from build123d import *

# Parameters (mm, degrees)
F0_W      = 1778
F0_H      = 279.4
F1_DEPTH  = 25.4
F2_W      = 1727.2
F2_H      = 228.6
F3_DEPTH  = 25.401
F4_W      = 279.4
F4_H      = 279.4
F5_DEPTH  = 25.4
F6_W      = 127
F6_H      = 25.4
F7_DEPTH  = 25.4
F8_W      = 127
F8_H      = 25.4
F9_DEPTH  = 25.4
F10_W     = 127
F10_H     = 25.4
F11_DEPTH = 25.4
F12_W     = 127
F12_H     = 25.4
F13_DEPTH = 25.4


with BuildPart() as f1:
    # F0 (on Top) → F1 (new body)
    with BuildSketch(Plane.XY):
        Rectangle(F0_W, F0_H)
    extrude(amount=F1_DEPTH)

    # F2 (on face) → F3 (cut, through all)
    with BuildSketch(Plane.XY.offset(25.4)):
        Rectangle(F2_W, F2_H)
    extrude(amount=-F3_DEPTH, mode=Mode.SUBTRACT)

    # F4 (on Top) → F5 (join)
    with BuildSketch(Plane.XY):
        Rectangle(F4_W, F4_H)
    extrude(amount=F5_DEPTH)

    # F6 (on face) → F7 (join)
    with BuildSketch(Plane(origin=(-889, 0, 0), x_dir=(0, -1, 0), z_dir=(-1, 0, 0))):
        with Locations((0, 12.7)):
            Rectangle(F6_W, F6_H)
    extrude(amount=F7_DEPTH)

    # F8 (on face) → F9 (join)
    with BuildSketch(Plane(origin=(863.6, 0, 0), x_dir=(0, -1, 0), z_dir=(-1, 0, 0))):
        with Locations((0, 12.7)):
            Rectangle(F8_W, F8_H)
    extrude(amount=F9_DEPTH)

    # F10 (on face) → F11 (join)
    with BuildSketch(Plane.YZ.offset(889)):
        with Locations((0, 12.7)):
            Rectangle(F10_W, F10_H)
    extrude(amount=F11_DEPTH)

    # F12 (on face) → F13 (join)
    with BuildSketch(Plane.YZ.offset(-863.6)):
        with Locations((0, 12.7)):
            Rectangle(F12_W, F12_H)
    extrude(amount=F13_DEPTH)


solid = f1.part
Verification items for the finished model (mm, model axes). Coordinates: 2 decimals unless noted, no trailing zeros. Order: outer loops, then holes, each group sorted by start corner. A loop starts at its lowest first (then second) coordinate and runs counter-clockwise, first axis right, second up. Notation, with made-up numbers: (31, -3.75) -> (89, -3.75) arc R15 ccw to (89, 9.25) -> close; hole circle Ø10 at (-21, -27). An arc over 180 degrees is marked (long way). Put each result on its own line as item: value. Start each with the question number.
1. Material ranges on L1, parallel to X at y = 79.5, z = 18.25; L2, parallel to X at y = -21.5, z = 5.25; L3, parallel to Y at x = 687, z = 19, recorded low to high. Write a range as [from, to].
2. Cross-section at A-A, the plane y = -43.5. Record the boundary of the cut face in (x, z), then the cut area to 3 significant figures.
3. Cross-section at B-B, the plane x = -739. Record the boundary of the cut face in (y, z).
4. Cross-section at C-C, the plane z = 17. Record the boundary of the cut face in (x, y).
5. Go/stop test with flat-tipped pins: pin 1 Ø7.5 at (y, z) = (94.5, 16) entering from +X; pin 2 Ø10 at (y, z) = (95, 12) entering from -X. Record where each tip stops, or that it passes through.
Computed:
1. L1: [-889, -863.6], [-139.7, 139.7], [863.6, 889]
1. L2: [-914.4, -838.2], [-139.7, 139.7], [838.2, 914.4]
1. L3: [-139.7, -114.3], [114.3, 139.7]
2. outline: (-914.4, 0) -> (-838.2, 0) -> (-838.2, 25.4) -> (-914.4, 25.4) -> close; (-139.7, 0) -> (139.7, 0) -> (139.7, 25.4) -> (-139.7, 25.4) -> close; (838.2, 0) -> (914.4, 0) -> (914.4, 25.4) -> (838.2, 25.4) -> close
2. area: 11,000 mm2
3. outline: (-139.7, 0) -> (-114.3, 0) -> (-114.3, 25.4) -> (-139.7, 25.4) -> close; (114.3, 0) -> (139.7, 0) -> (139.7, 25.4) -> (114.3, 25.4) -> close
4. outline: (-914.4, -63.5) -> (-889, -63.5) -> (-889, -139.7) -> (889, -139.7) -> (889, -63.5) -> (914.4, -63.5) -> (914.4, 63.5) -> (889, 63.5) -> (889, 139.7) -> (-889, 139.7) -> (-889, 63.5) -> (-914.4, 63.5) -> close; hole (-863.6, -114.3) -> (-139.7, -114.3) -> (-139.7, 114.3) -> (-863.6, 114.3) -> (-863.6, 63.5) -> (-838.2, 63.5) -> (-838.2, -63.5) -> (-863.6, -63.5) -> close; hole (139.7, -114.3) -> (863.6, -114.3) -> (863.6, -63.5) -> (838.2, -63.5) -> (838.2, 63.5) -> (863.6, 63.5) -> (863.6, 114.3) -> (139.7, 114.3) -> close
5. pin 1: x = 889
5. pin 2: x = -889
